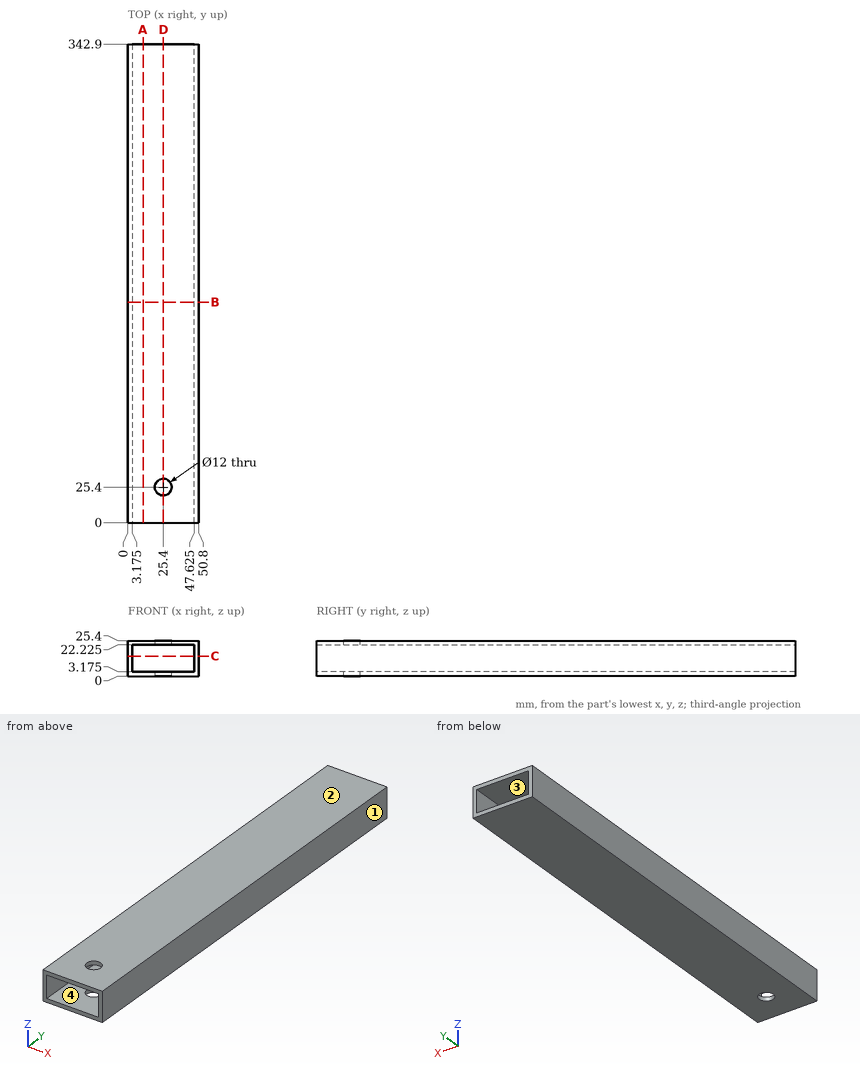
Could you check a few things on this drawing? It's one solid part, dimensions in mm from its lowest x, y, z. Give positions to 0.01 mm unless a question says otherwise; leave off trailing zeros. Order: outer loops, then holes, each group sorted by start corner. A loop starts at its lowest first (then second) coordinate and runs counter-clockwise, first axis right, second up. Notation, with made-up numbers: (-38.75, 52) - (14.25, 52) arc R19 cw to (14.25, 86) - close; hole circle Ø1 at (38, 15.5). An arc over 180 degrees is marked (long way). Return JSON: item names as keys, results as strings. Group by question number.
Q1. Suppose I cut it at A-A, the plane x = 11. Please give me the cut outline in (y, z) (3 decimals).
Q2. Suppose I cut it at C-C, the plane z = 14.25. Please give me the cut outline in (x, y) (3 decimals), and give its area (3 significant figures).
Q3. Suppose I cut it at D-D, the plane x = 25.5. Please give me the cut outline in (y, z) (3 decimals).
Q4. Thinking about a two-plate mould opening in Z: for the marked faces 1, 2, 3 and 4, which applies, pulls with the +Z half, pulls with the -Z half, needs draft (parallel to the pull), parting line crosses it, or undercut?
Q5. Suppose I cut it at B-B, the plane y = 158. Please give me the cut outline in (x, z) (3 decimals), and give its area (3 significant figures).
Q6. Will this pin go through, and if not, where does the flat tip stop? pin 1 Ø15 at (y, z) = (256, 15) entering from -X.
Q7. Please list where these lines run through material, in increasing order: line 1 along X through (y, z) = (25.4, 2.2); line 2 along X through (y, z) = (247.5, 17.25) (3 decimals); line 3 along Y through (x, z) = (25.4, 1.95). Write a range as [from, to].
Resolved:
{
 "1": {"outline": "(0, 0) - (342.9, 0) - (342.9, 3.175) - (0, 3.175) - close; (0, 22.225) - (342.9, 22.225) - (342.9, 25.4) - (0, 25.4) - close"},
 "2": {"outline": "(0, 0) - (3.175, 0) - (3.175, 342.9) - (0, 342.9) - close; (47.625, 0) - (50.8, 0) - (50.8, 342.9) - (47.625, 342.9) - close", "area": "2,180 mm2"},
 "3": {"outline": "(0, 0) - (19.401, 0) - (19.401, 3.175) - (0, 3.175) - close; (0, 22.225) - (19.401, 22.225) - (19.401, 25.4) - (0, 25.4) - close; (31.399, 0) - (342.9, 0) - (342.9, 3.175) - (31.399, 3.175) - close; (31.399, 22.225) - (342.9, 22.225) - (342.9, 25.4) - (31.399, 25.4) - close"},
 "4": {"face 1": "needs draft", "face 2": "pulls with the +Z half", "face 3": "undercut", "face 4": "undercut"},
 "5": {"outline": "(0, 0) - (50.8, 0) - (50.8, 25.4) - (0, 25.4) - close; hole (3.175, 3.175) - (47.625, 3.175) - (47.625, 22.225) - (3.175, 22.225) - close", "area": "444 mm2"},
 "6": {"pin 1": "stops at x = 0"},
 "7": {"line 1": "x = [0, 19.4], [31.4, 50.8]", "line 2": "x = [0, 3.175], [47.625, 50.8]", "line 3": "y = [0, 19.4], [31.4, 342.9]"}
}
